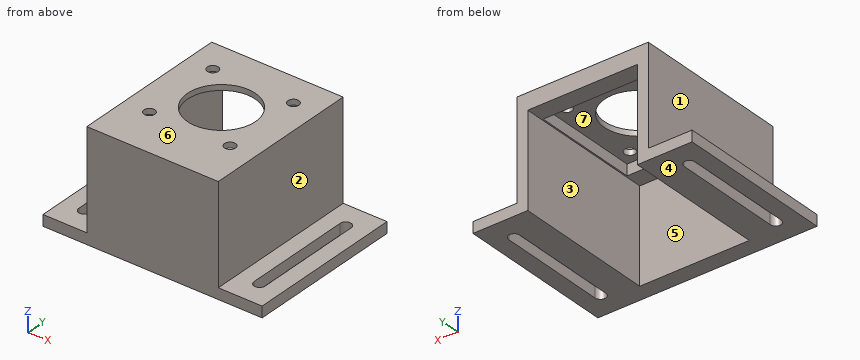
```python
from build123d import *

# Parameters (mm, degrees)
SKETCH2_W           = 76.2
SKETCH2_H           = 63.5
BOSS_EXTRUDE1_DEPTH = 9.525
SKETCH3_W           = 76.2
SKETCH3_H           = 9.525
BOSS_EXTRUDE2_DEPTH = 82.55
SKETCH7_R           = 19.685
SKETCH7_R_2         = 3.175
CUT_EXTRUDE1_DEPTH  = 10.525
SKETCH11_W          = 61.921486798
SKETCH11_H          = 61.884587426
CUT_EXTRUDE4_DEPTH  = 6.35
SKETCH12_W          = 6.35
SKETCH12_H          = 53.975
BOSS_EXTRUDE3_DEPTH = 82.55
SKETCH14_W          = 6.35
SKETCH14_H          = 92.075
BOSS_EXTRUDE5_DEPTH = 25.4
SKETCH15_W          = 6.35
SKETCH15_H          = 92.075
BOSS_EXTRUDE6_DEPTH = 25.4
CUT_EXTRUDE5_DEPTH  = 7.35


with BuildPart() as part:
    # Sketch2 → Boss-Extrude1 (new body)
    with BuildSketch(Plane(origin=(0, 0, 0), x_dir=(1, 0, 0), z_dir=(0, 1, 0))):
        with Locations((38.1, 31.75)):
            Rectangle(SKETCH2_W, SKETCH2_H)
    extrude(amount=BOSS_EXTRUDE1_DEPTH)

    # Sketch3 → Boss-Extrude2 (add)
    with BuildSketch(Plane(origin=(0, 9.525, 0), x_dir=(1, 0, 0), z_dir=(0, 1, 0))):
        with Locations((38.1, 4.7625)):
            Rectangle(SKETCH3_W, SKETCH3_H)
    extrude(amount=BOSS_EXTRUDE2_DEPTH)

    # Sketch7 → Cut-Extrude1 (cut, through all)
    with BuildSketch(Plane(origin=(0, 0, -9.525), x_dir=(-1, 0, 0), z_dir=(0, 0, -1))):
        with Locations((-38.1, 50.8)):
            Circle(SKETCH7_R)
        with Locations((-61.468, 74.168)):
            Circle(SKETCH7_R_2)
        with Locations((-14.732, 74.168)):
            Circle(SKETCH7_R_2)
        with Locations((-14.732, 27.432)):
            Circle(SKETCH7_R_2)
        with Locations((-61.468, 27.432)):
            Circle(SKETCH7_R_2)
    extrude(amount=-CUT_EXTRUDE1_DEPTH, mode=Mode.SUBTRACT)

    # Sketch11 → Cut-Extrude4 (cut)
    with BuildSketch(Plane(origin=(0, 0, -9.525), x_dir=(-1, 0, 0), z_dir=(0, 0, -1))):
        with Locations((-38.1, 50.8)):
            Rectangle(SKETCH11_W, SKETCH11_H)
    extrude(amount=-CUT_EXTRUDE4_DEPTH, mode=Mode.SUBTRACT)

    # Sketch12 → Boss-Extrude3 (add)
    with BuildSketch(Plane(origin=(0, 9.525, 0), x_dir=(1, 0, 0), z_dir=(0, 1, 0))):
        with Locations((73.025, 36.5125)):
            Rectangle(SKETCH12_W, SKETCH12_H)
        with Locations((3.175, 36.5125)):
            Rectangle(SKETCH12_W, SKETCH12_H)
    extrude(amount=BOSS_EXTRUDE3_DEPTH)

    # Sketch14 → Boss-Extrude5 (add)
    with BuildSketch(Plane.ZY):
        with Locations((-60.325, 46.0375)):
            Rectangle(SKETCH14_W, SKETCH14_H)
    extrude(amount=BOSS_EXTRUDE5_DEPTH)

    # Sketch15 → Boss-Extrude6 (add)
    with BuildSketch(Plane(origin=(76.2, 0, 0), x_dir=(0, 0, -1), z_dir=(1, 0, 0))):
        with Locations((60.325, 46.0375)):
            Rectangle(SKETCH15_W, SKETCH15_H)
    extrude(amount=BOSS_EXTRUDE6_DEPTH)

    # Sketch16 → Cut-Extrude5 (cut, through all)
    with BuildSketch(Plane.XY.offset(-57.15)):
        with BuildLine():
            Line((-15.875, 77.7875), (-15.875, 14.2875))
            ThreePointArc((-15.875, 14.2875), (-12.7, 11.1125), (-9.525, 14.2875))
            Line((-9.525, 14.2875), (-9.525, 77.7875))
            ThreePointArc((-9.525, 77.7875), (-12.7, 80.9625), (-15.875, 77.7875))
        make_face()
        with BuildLine():
            Line((85.725, 14.2875), (85.725, 77.7875))
            ThreePointArc((85.725, 77.7875), (88.9, 80.9625), (92.075, 77.7875))
            Line((92.075, 77.7875), (92.075, 14.2875))
            ThreePointArc((92.075, 14.2875), (88.9, 11.1125), (85.725, 14.2875))
        make_face()
    extrude(amount=-CUT_EXTRUDE5_DEPTH, mode=Mode.SUBTRACT)


solid = part.part
```
Input: part model. Units: mm. Frame: model coordinates. Face numbers are marked on the shaded views. A direction names the side the tool comes from. Coordinates: 2 decimals unless noted, no trailing zeros. Write each loop counter-clockwise with the first axis right and the second up, starting at its lowest first coordinate (ties: lowest second). Pieces come first, ordered by that corner, then holes.
1) Material intervals for line 1 along X through (y, z) = (78.5, -56); line 2 along X through (y, z) = (24, -6); line 3 along Z through (x, y) = (-10.5, 85), sorted ascending.
2) Pin query (flat end, axial travel): pin 1 Ø8 at (y, z) = (30.5, -13.5) entering from -X; pin 2 Ø12 at (x, z) = (49, -30) entering from -Y; pin 3 Ø12 at (y, z) = (24.5, -6.5) entering from +X; pin 4 Ø10 at (x, y) = (61.468, 74.168) entering from -Z (3 decimals). Return the tip coordinate at first contact, or that it passes through.
3) Section A-A on x = 38.1. Output: boundary loops of the cut face in (y, z) (3 decimals).
4) Section C-C on y = 52.5. Output: boundary loops of the cut face in (x, z) (3 decimals), and give its area (3 significant figures).
5) Set-up query: the marked faces 1, 2, 3 and 4. Return all of +Z, -Z, +X, -X, +Y, -Y with unobstructed straight access to the full face (end or side cutting, diameter ignored); none if empty.
6) Section B-B on z = -7. Output: boundary loops of the cut face in (x, y) (3 decimals).
7) Mould query, pull axis Z, two halves, no side actions, for the marked faces 5, 6 and 7. Classes: pulls with the +Z half, pulls with the -Z half, needs draft (parallel to the pull), parting line crosses it, or undercut.
Check result:
1. line 1: x = 0 to 6.35, 69.85 to 76.2
1. line 2: x = 0 to 7.14, 69.06 to 76.2
1. line 3: z = -63.5 to -57.15
2. pin 1: stops at x = 0
2. pin 2: stops at y = 0
2. pin 3: stops at x = 76.2
2. pin 4: stops at z = -3.175
3. outline: (0, -63.5) - (9.525, -63.5) - (9.525, -9.525) - (19.858, -9.525) - (19.858, -3.175) - (31.115, -3.175) - (31.115, 0) - (0, 0) - close; (70.485, -3.175) - (81.742, -3.175) - (81.742, -9.525) - (92.075, -9.525) - (92.075, 0) - (70.485, 0) - close
4. outline: (-25.4, -63.5) - (-15.875, -63.5) - (-15.875, -57.15) - (-25.4, -57.15) - close; (-9.525, -63.5) - (6.35, -63.5) - (6.35, -9.525) - (7.139, -9.525) - (7.139, -3.175) - (18.489, -3.175) - (18.489, 0) - (0, 0) - (0, -57.15) - (-9.525, -57.15) - close; (57.711, -3.175) - (69.061, -3.175) - (69.061, -9.525) - (69.85, -9.525) - (69.85, -63.5) - (85.725, -63.5) - (85.725, -57.15) - (76.2, -57.15) - (76.2, 0) - (57.711, 0) - close; (92.075, -63.5) - (101.6, -63.5) - (101.6, -57.15) - (92.075, -57.15) - close
4. area: 1,140 mm2
5. face 1: +Z, -X, +Y, -Y
5. face 2: +Z, +X, +Y, -Y
5. face 3: -Z, +Y
5. face 4: -Z, +X, -X, +Y, -Y
6. outline: (0, 0) - (76.2, 0) - (76.2, 92.075) - (0, 92.075) - close; hole (7.139, 19.858) - (69.061, 19.858) - (69.061, 81.742) - (7.139, 81.742) - close
7. face 5: needs draft
7. face 6: pulls with the +Z half
7. face 7: pulls with the -Z half
